```python
from build123d import *

# Parameters (mm, degrees)
ESQUISSE2_R             = 24.5
ENL_V_MAT_EXTRU_1_DEPTH = 10
ESQUISSE4_R             = 14
ENL_V_MAT_EXTRU_2_DEPTH = 97.42095208
ESQUISSE5_R             = 15
ENL_V_MAT_EXTRU_3_DEPTH = 20
ENL_V_START             = -20
ESQUISSE6_R             = 15
ENL_V_MAT_EXTRU_4_DEPTH = 20


with BuildPart() as part:
    # Esquisse1 → Révolution1 (revolve)
    with BuildSketch(Plane.XY, mode=Mode.PRIVATE) as r_volution1_sk:
        Polygon((0, 0), (0, 35), (5, 35), (5, 55), (6, 56), (14, 56), (14, 0), align=None)
    revolve(r_volution1_sk.sketch.rotate(Axis((0, 0, 0), (1, 0, 0)), 90), axis=Axis((0, 0, 0), (1, 0, 0)))

    # Esquisse2 → Enlèv. mat.-Extru.1 (cut)
    with BuildSketch(Plane.ZY):
        Circle(ESQUISSE2_R)
    extrude(amount=-ENL_V_MAT_EXTRU_1_DEPTH, mode=Mode.SUBTRACT)

    # Esquisse3 → Révolution2 (revolve)
    with BuildSketch(Plane.XY):
        Polygon((14, 21), (17, 21), (17, 18), (59, 18), (59, 17), (61, 17), (61, 18), (65, 18), (65, -9), (14, -9), align=None)
    revolve(axis=Axis((58.599942934, -9, 0), (-1, 0, 0)))

    # Esquisse4 → Enlèv. mat.-Extru.2 (cut, through all)
    with BuildSketch(Plane.ZY.offset(-10)):
        Circle(ESQUISSE4_R)
    extrude(amount=-ENL_V_MAT_EXTRU_2_DEPTH, mode=Mode.SUBTRACT)

    # Esquisse5 → Enlèv. mat.-Extru.3 (cut)
    with BuildSketch(Plane.ZY.offset(-10)):
        Circle(ESQUISSE5_R)
    extrude(amount=-ENL_V_MAT_EXTRU_3_DEPTH, mode=Mode.SUBTRACT)

    # Esquisse6 → Enlèv. mat.-Extru.4 (cut)
    with BuildSketch(Plane(origin=(65, 0, 0), x_dir=(0, 0, -1), z_dir=(1, 0, 0)).offset(ENL_V_START)):
        with Locations(Location((0, 0, 0), (0, 0, 180))):
            Circle(ESQUISSE6_R)
    extrude(amount=ENL_V_MAT_EXTRU_4_DEPTH, mode=Mode.SUBTRACT)


solid = part.part
```
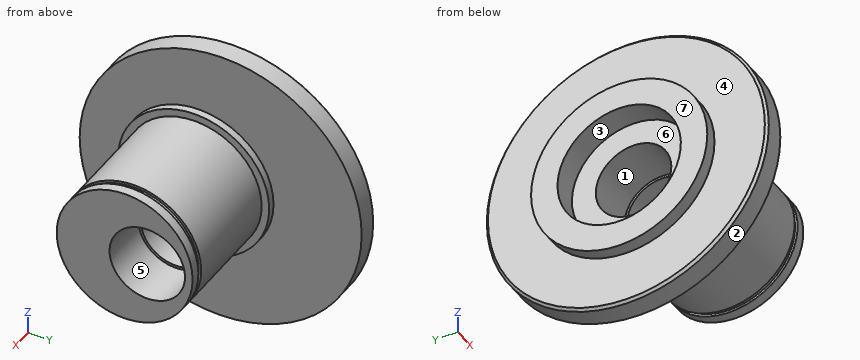
The model under review builds one solid part; all positions refer to its coordinate system, in mm. Face numbers are marked on the shaded views. A direction names the side the tool comes from. Give positions to 0.01 mm unless a question says otherwise; leave off trailing zeros. Write each loop counter-clockwise with the first axis right and the second up, starting at its lowest first coordinate (ties: lowest second). Pieces come first, ordered by that corner, then holes. Notation, with made-up numbers: M 34.25,18 L 52.25,18 A16 cw 52.25,29 Z; hole C 29,80.5 d4. An arc over 180 degrees is marked long. Answer in a Markdown table with one row per item.
Item 1: For P1, Ø4, axis at x = 18.5, z = -1, coming from the +Y side; P2, Ø2, axis at x = 30.5, y = -8.5, coming from the +Z side; P3, Ø12, axis at y = -40.5, z = -17.5, coming from the -X side, all flat-tipped, find the tip position at first contact; note any pin that passes through.
Check sheet entries:
| item | result |
|---|---|
| P1 | y = 21 |
| P2 | z = 27 |
| P3 | x = 5 |
Item 2: For line 1 along Y through (x, z) = (56, 0); line 2 along Y through (x, z) = (15.75, 0); line 3 along X through (y, z) = (0.5, -43.5), list the stretches that pass through material, from the lowest coordinate up.
Check sheet entries:
| item | result |
|---|---|
| line 1 | -36 to -15, 15 to 18 |
| line 2 | -39 to -15, 15 to 21 |
| line 3 | 5 to 14 |
Item 3: Add section A-A on x = 21.5. Give the boundary of the cut face in (y, z).
Check sheet entries:
| item | result |
|---|---|
| outline | C -9,0 d54; hole C 0,0 d30 |
Item 4: Draft analysis for pull direction Y (two halves, no side actions). For the marked faces 1, 2, 3 and 4, state which applies: +Y half, -Y half, draft (parallel to the pull), parting line (faces both ways), or undercut.
Check sheet entries:
| item | result |
|---|---|
| face 1 | undercut |
| face 2 | parting line |
| face 3 | undercut |
| face 4 | draft |
Item 5: Tool access review of the marked faces 5, 6 and 7: name each direction out of +Z, -Z, +X, -X, +Y, -Y from which nothing blocks a thin tool from reaching the whole face with its end or side.
Check sheet entries:
| item | result |
|---|---|
| face 5 | +X |
| face 6 | -X |
| face 7 | +Z, -Z, -X, +Y, -Y |
